```python
from build123d import *

# Parameters (mm, degrees)
SKETCH4_R           = 3.190875
BOSS_EXTRUDE1_DEPTH = 7.14375
SKETCH5_OUTSIDE_W   = 72.142
SKETCH5_OUTSIDE_H   = 70.914
SKETCH5_OUTSIDE_R   = 3.86953125
CUT_EXTRUDE1_DEPTH  = 16.520468256
CUT_EXTRUDE1_DRAFT  = -60
SKETCH6_OUTSIDE_W   = 72.142
SKETCH6_OUTSIDE_H   = 70.914
SKETCH6_OUTSIDE_R   = 3.86953125
CUT_EXTRUDE2_DEPTH  = 16.520468256
CUT_EXTRUDE2_DRAFT  = -60
FILLET1_R           = 0.79375


with BuildPart() as part:
    # Sketch3 → Revolve1 (revolve)
    with BuildSketch(Plane(origin=(0, 0, 0), x_dir=(0, 0, -1), z_dir=(1, 0, 0)), mode=Mode.PRIVATE) as revolve1_sk:
        Polygon((7.14375, 2.6114375), (7.14375, 3.96875), (0, 3.96875), (-7.14375, 3.96875), (-7.14375, 2.6114375), (-6.9453125, 2.413), (6.9453125, 2.413), align=None)
        Polygon((7.14375, 2.6114375), (7.14375, 3.96875), (0, 3.96875), (-7.14375, 3.96875), (-7.14375, 2.6114375), (-6.9453125, 2.413), (6.9453125, 2.413), align=None)
    revolve(revolve1_sk.sketch.rotate(Axis((0, 0, -7.14375), (0, 0, 1)), 90), axis=Axis((0, 0, -7.14375), (0, 0, 1)))

    # Sketch4 → Boss-Extrude1 (add, symmetric)
    with BuildSketch(Plane.XY):
        Polygon((-2.291358881, 3.96875), (-4.582717762, 0), (-2.291358881, -3.96875), (2.291358881, -3.96875), (4.582717762, 0), (2.291358881, 3.96875), align=None)
        Circle(SKETCH4_R, mode=Mode.SUBTRACT)
    extrude(amount=BOSS_EXTRUDE1_DEPTH, both=True)


with BuildPart() as cut_extrude1_tool:
    # Sketch5 outside → Cut-Extrude1 (with draft: the straight prism first)
    with BuildSketch(Plane.XY.offset(7.14375)):
        Rectangle(SKETCH5_OUTSIDE_W, SKETCH5_OUTSIDE_H)
        Circle(SKETCH5_OUTSIDE_R, mode=Mode.SUBTRACT)
    extrude(amount=-CUT_EXTRUDE1_DEPTH)
    # Cut-Extrude1: the draft: its side faces are tilted about the plane it starts from
    cut_extrude1_sides = [cut_extrude1_tool.faces().sort_by_distance(p)[0] for p in [
        (0, -35.457, -1.116484128),
        (36.071, 0, -1.116484128),
        (0, 35.457, -1.116484128),
        (-36.071, 0, -1.116484128),
        (-3.86953125, 0, -1.116484128),
    ]]
    draft(cut_extrude1_sides, Plane.XY.offset(7.14375), CUT_EXTRUDE1_DRAFT)


with BuildPart() as part_1:
    add(part.part)

    # Cut-Extrude1: cut by cut_extrude1_tool
    add(cut_extrude1_tool.part, mode=Mode.SUBTRACT)


with BuildPart() as cut_extrude2_tool:
    # Sketch6 outside → Cut-Extrude2 (with draft: the straight prism first)
    with BuildSketch(Plane(origin=(0, 0, -7.14375), x_dir=(-1, 0, 0), z_dir=(0, 0, -1))):
        Rectangle(SKETCH6_OUTSIDE_W, SKETCH6_OUTSIDE_H)
        Circle(SKETCH6_OUTSIDE_R, mode=Mode.SUBTRACT)
    extrude(amount=-CUT_EXTRUDE2_DEPTH)
    # Cut-Extrude2: the draft: its side faces are tilted about the plane it starts from
    cut_extrude2_sides = [cut_extrude2_tool.faces().sort_by_distance(p)[0] for p in [
        (0, -35.457, 1.116484128),
        (-36.071, 0, 1.116484128),
        (0, 35.457, 1.116484128),
        (36.071, 0, 1.116484128),
        (3.86953125, 0, 1.116484128),
    ]]
    draft(cut_extrude2_sides, Plane(origin=(0, 0, -7.14375), x_dir=(-1, 0, 0), z_dir=(0, 0, -1)), CUT_EXTRUDE2_DRAFT)


with BuildPart() as part_2:
    add(part_1.part)

    # Cut-Extrude2: cut by cut_extrude2_tool
    add(cut_extrude2_tool.part, mode=Mode.SUBTRACT)

    # Fillet1
    # the kernel refuses this fillet: 0.79375 mm, written as the material it takes off along each edge
    with BuildSketch(Plane(origin=(2.291358881, 3.96875, 7.877671016), x_dir=(0.49999999999999933, -0.866025403784439, 0), z_dir=(0, 0, -1)), Plane(origin=(-4.582717762, 0, -7.877671016), x_dir=(0.5000000000000004, -0.8660254037844384, 0), z_dir=(0, 0, 1)), Plane(origin=(4.582717762, 0, 7.877671016), x_dir=(-0.49999999999999917, -0.8660254037844392, 0), z_dir=(0, 0, -1)), Plane(origin=(-2.291358881, 3.96875, 7.877671016), x_dir=(1, 0, 0), z_dir=(0, 0, -1))) as fillet1_piece_1:
        with BuildLine():
            CenterArc((FILLET1_R * 0.57735026919, FILLET1_R), FILLET1_R, 210, 60)
            Line((-FILLET1_R * 0.288675134595, FILLET1_R * 0.5), (0, 0))
            Line((0, 0), (FILLET1_R * 0.57735026919, 0))
        make_face()
    extrude(amount=15.755342032, mode=Mode.SUBTRACT)
    with BuildSketch(Plane(origin=(-2.291358881, -3.96875, -7.877671016), x_dir=(-0.5000000000000001, 0.8660254037844386, 0), z_dir=(0, 0, 1)), Plane(origin=(2.291358881, -3.96875, -7.877671016), x_dir=(-1, 0, 0), z_dir=(0, 0, 1))) as fillet1_piece_2:
        with BuildLine():
            CenterArc((FILLET1_R * 0.57735026919, -FILLET1_R), FILLET1_R, 90, 60)
            Line((-FILLET1_R * 0.288675134595, -FILLET1_R * 0.5), (0, 0))
            Line((0, 0), (FILLET1_R * 0.57735026919, 0))
        make_face()
    extrude(amount=15.755342032, mode=Mode.SUBTRACT)


solid = part_2.part
```
Read the model definition and answer for the solid it produces. Units are mm, in the model's axes. Give positions to 0.01 mm unless a question says otherwise; leave off trailing zeros. Order: outer loops, then holes, each group sorted by start corner. A loop starts at its lowest first (then second) coordinate and runs counter-clockwise, first axis right, second up.
(1) Straight lines are drawn through the part: L1, parallel to Y at x = 0, z = -2.25; L2, parallel to X at y = 1.25, z = -1.5; L3, parallel to X at y = -1.5, z = -6.5. For each, find the intervals that lie inside material, in ascending order.
(2) Find section A-A (x = 0). Give the vertices of the cut face in (y, z).
(3) For a pull along X with two mould halves and no side action, classify faces 1 (the flat face through (0, 3.969, 0)), 2 (the flat face through (-3.45, -1.96, 0.1)), 3 (the cylindrical face through (1.915, 1.468, -0.097)) as released by +X, released by -X, zero draft, split by the parting line, or undercut.
(4) Find section C-C (y = 0). Give the vertices of the cut face in (x, z).
(5) Given pin 1 (4 mm diameter, centred on x = 0, y = 0, fed in from -Z); pin 2 (3 mm diameter, centred on y = 2, z = 4.5, fed in from +X), each flat-ended and moving along its own axis, determine where each tip first touches the part or whether it passes through.
(6) Find section B-B (z = -2.75). Give the vertices of the cut face in (x, y) (1 decimal).
Result sheet:
1. L1: y = -3.97 to -2.41, 2.41 to 3.97
1. L2: x = -3.86 to -2.06, 2.06 to 3.86
1. L3: x = -3.72 to -1.89, 1.89 to 3.72
2. outline: (-3.97, -7.09) - (-3.87, -7.14) - (-2.61, -7.14) - (-2.41, -6.95) - (-2.41, 6.95) - (-2.61, 7.14) - (-3.87, 7.14) - (-3.97, 7.09) - close; (2.41, -6.95) - (2.61, -7.14) - (3.87, -7.14) - (3.97, -7.09) - (3.97, 7.09) - (3.87, 7.14) - (2.61, 7.14) - (2.41, 6.95) - close
3. face 1: zero draft
3. face 2: released by -X
3. face 3: undercut
4. outline: (-4.46, -6.8) - (-3.87, -7.14) - (-2.61, -7.14) - (-2.41, -6.95) - (-2.41, 6.95) - (-2.61, 7.14) - (-3.87, 7.14) - (-4.46, 6.8) - close; (2.41, -6.95) - (2.61, -7.14) - (3.87, -7.14) - (4.46, -6.8) - (4.46, 6.8) - (3.87, 7.14) - (2.61, 7.14) - (2.41, 6.95) - close
5. pin 1: passes through
5. pin 2: stops at x = 4.29
6. outline: (-4.4, -0.4) - (-2.5, -3.6) arc R0.8 ccw to (-1.8, -4) - (1.8, -4) arc R0.8 ccw to (2.5, -3.6) - (4.4, -0.4) arc R0.8 ccw to (4.4, 0.4) - (2.5, 3.6) arc R0.8 ccw to (1.8, 4) - (-1.8, 4) arc R0.8 ccw to (-2.5, 3.6) - (-4.4, 0.4) arc R0.8 ccw to start; hole circle Ø4.8 at (0, 0)
